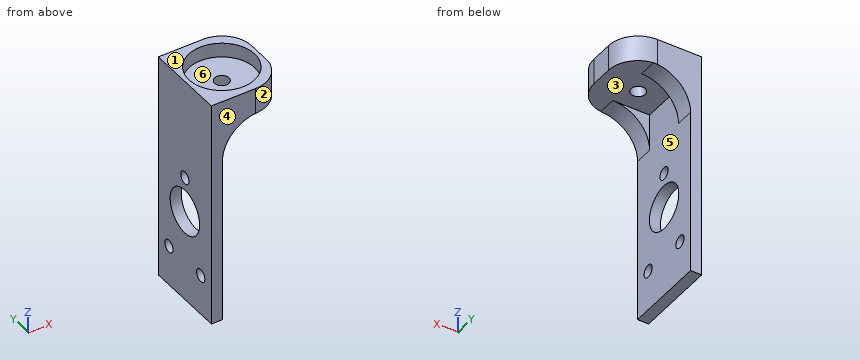
```python
from build123d import *

# Parameters (mm, degrees)
SKETCH1_W                 = 3.81
SKETCH1_H                 = 78.74
SKETCH1_W_2               = 21.59
SKETCH1_H_2               = 8.89
BOSS_EXTRUDE1_DEPTH       = 27.94
SKETCH2_R                 = 11.303
CUT_EXTRUDE1_DEPTH        = 4.953
F_8_CLEARANCE_HOLE1_D     = 4.9149
CUT_EXTRUDE4_REACH        = 88.295
SKETCH5_R                 = 7.747
F_6_CLEARANCE_HOLE1_D     = 4.3053
F_6_CLEARANCE_HOLE1_DEPTH = 3.81
FILLET1_DEPTH             = 6.35
FILLET2_START             = 21.59
FILLET2_DEPTH             = 6.35
FILLET3_R                 = 10.16


with BuildPart() as part:
    # Sketch1 → Boss-Extrude1 (new body)
    with BuildSketch(Plane(origin=(0, 0, 0), x_dir=(1, 0, 0), z_dir=(0, 1, 0))):
        with Locations((1.905, 39.37)):
            Rectangle(SKETCH1_W, SKETCH1_H)
        with Locations((14.605, 4.445)):
            Rectangle(SKETCH1_W_2, SKETCH1_H_2)
    extrude(amount=BOSS_EXTRUDE1_DEPTH)

    # Sketch2 → Cut-Extrude1 (cut)
    with BuildSketch(Plane.XY):
        with Locations((12.7, 13.97)):
            Circle(SKETCH2_R)
    extrude(amount=-CUT_EXTRUDE1_DEPTH, mode=Mode.SUBTRACT)

    # #8 Clearance Hole1 (through all)
    with Locations(Plane.XY.offset(-4.953)):
        with Locations((12.7, 13.97)):
            Hole(F_8_CLEARANCE_HOLE1_D / 2)

    # Sketch5 → Cut-Extrude4 (cut, up to next)
    with BuildSketch(Plane(origin=(3.81, 0, 0), x_dir=(0, 0, -1), z_dir=(1, 0, 0)), mode=Mode.PRIVATE) as cut_extrude4_sk1:
        with Locations((46.99, 13.97)):
            Circle(SKETCH5_R)
    cut_extrude4_tool1 = extrude(cut_extrude4_sk1.sketch, amount=-CUT_EXTRUDE4_REACH, mode=Mode.PRIVATE) & part.part
    # Sketch5 → Cut-Extrude4 (cut, up to next)
    with BuildSketch(Plane(origin=(3.81, 0, 0), x_dir=(0, 0, -1), z_dir=(1, 0, 0)), mode=Mode.PRIVATE) as cut_extrude4_sk2:
        with BuildLine():
            ThreePointArc((54.737, 13.97), (46.99, 21.717), (39.243, 13.97))
            Line((39.243, 13.97), (54.737, 13.97))
        make_face()
    cut_extrude4_tool2 = extrude(cut_extrude4_sk2.sketch, amount=-CUT_EXTRUDE4_REACH, mode=Mode.PRIVATE) & part.part
    # Sketch5 → Cut-Extrude4 (cut, up to next)
    with BuildSketch(Plane(origin=(3.81, 0, 0), x_dir=(0, 0, -1), z_dir=(1, 0, 0)), mode=Mode.PRIVATE) as cut_extrude4_sk3:
        with BuildLine():
            Line((54.737, 13.97), (39.243, 13.97))
            ThreePointArc((39.243, 13.97), (46.99, 6.223), (54.737, 13.97))
        make_face()
    cut_extrude4_tool3 = extrude(cut_extrude4_sk3.sketch, amount=-CUT_EXTRUDE4_REACH, mode=Mode.PRIVATE) & part.part
    add(cut_extrude4_tool1.solids().sort_by_distance((3.81, 13.97, -46.99))[0], mode=Mode.SUBTRACT)
    add(cut_extrude4_tool2.solids().sort_by_distance((3.81, 17.257929, -46.99))[0], mode=Mode.SUBTRACT)
    add(cut_extrude4_tool3.solids().sort_by_distance((3.81, 10.682071, -46.99))[0], mode=Mode.SUBTRACT)

    # #6 Clearance Hole1
    with Locations(Plane(origin=(3.81, 0, 0), x_dir=(0, 0, -1), z_dir=(1, 0, 0))):
        with Locations((34.798, 13.97), (46.99, 13.97), (64.77, 22.352), (64.77, 5.588)):
            Hole(F_6_CLEARANCE_HOLE1_D / 2, depth=F_6_CLEARANCE_HOLE1_DEPTH)

    # Fillet1: read off the stored shape, not the designer's step
    # Fillet1 outline → Fillet1 (add)
    with BuildSketch(Plane(origin=(0, 0, 0), x_dir=(1, 0, 0), z_dir=(0, 1, 0))):
        with BuildLine():
            ThreePointArc((16.51, 8.89), (7.529743879, 12.609743879), (3.81, 21.59))
            Line((3.81, 21.59), (3.81, 8.89))
            Line((3.81, 8.89), (16.51, 8.89))
        make_face()
    extrude(amount=FILLET1_DEPTH)

    # Fillet2: read off the stored shape, not the designer's step
    # Fillet2 outline → Fillet2 (add)
    with BuildSketch(Plane(origin=(0, 0, 0), x_dir=(1, 0, 0), z_dir=(0, 1, 0)).offset(FILLET2_START)):
        with BuildLine():
            ThreePointArc((16.51, 8.89), (7.529743879, 12.609743879), (3.81, 21.59))
            Line((3.81, 21.59), (3.81, 8.89))
            Line((3.81, 8.89), (16.51, 8.89))
        make_face()
    extrude(amount=FILLET2_DEPTH)

    # Fillet3
    fillet3_edges = [part.edges().sort_by_distance(p)[0] for p in [
        (25.4, 0, -4.445),
        (25.4, 27.94, -4.445),
    ]]
    fillet(fillet3_edges, radius=FILLET3_R)


solid = part.part
```
Can you work these out from the model? Positions are in its coordinate system, mm. Face numbers are marked on the shaded views. A direction names the side the tool comes from. Give positions to 0.01 mm unless a question says otherwise; leave off trailing zeros. Write each loop counter-clockwise with the first axis right and the second up, starting at its lowest first coordinate (ties: lowest second). Pieces come first, ordered by that corner, then holes. Notation, with made-up numbers: (20, -17.5) -> (39, -17.5) arc R20 ccw to (39, -6.5) -> close; hole circle Ø1 at (62.5, 49). An arc over 180 degrees is marked (long way). One line per item, written item: value.
Q1. Imagine slicing it at D-D on x = 14. Please give me the cut outline in (y, z).
Results found:
outline: (0, -9.14) -> (6.35, -9.14) -> (6.35, -8.89) -> (11.88, -8.89) -> (11.88, -4.95) -> (2.74, -4.95) -> (2.74, 0) -> (0, 0) -> close; (16.06, -8.89) -> (21.59, -8.89) -> (21.59, -9.14) -> (27.94, -9.14) -> (27.94, 0) -> (25.2, 0) -> (25.2, -4.95) -> (16.06, -4.95) -> close
Q2. Please list where these lines run through material, in increasing order: line 1 (Y direction, x = 2.55, z = -64.77); line 2 (Z direction, x = 3.75, y = 14.75); line 3 (X direction, y = 26.5, z = -65). Write a range as [from, to].
Results found:
line 1: y = [0, 3.44], [7.74, 20.2], [24.5, 27.94]
line 2: z = [-78.74, -54.7], [-39.28, -36.8], [-32.79, -4.95]
line 3: x = [0, 3.81]
Q3. Imagine slicing it at B-B on z = -46.99. Please give me the cut outline in (x, y).
Results found:
outline: (0, 0) -> (3.81, 0) -> (3.81, 6.22) -> (0, 6.22) -> close; (0, 21.72) -> (3.81, 21.72) -> (3.81, 27.94) -> (0, 27.94) -> close
Q4. For P1, Ø10, axis at x = 8.5, z = -16.5, coming from the +Y side; P2, Ø11.5, axis at x = 14, y = 11, coming from the +Z side; P3, Ø11, axis at x = 11.5, y = 17, coming from the -Z side, each with a flat end and sliding along its axis, tell me the tip position at first contact or that it passes through.
Results found:
P1: stops at y = 27.94
P2: stops at z = -4.95
P3: stops at z = -11.76
Q5. We'd pull the mould along Y, two halves only. Please class the marked faces 1, 2 and 3: +Y half, -Y half, draft (parallel to the pull), parting line (faces both ways), or undercut.
Results found:
face 1: draft
face 2: -Y half
face 3: undercut
Q6. Imagine slicing it at A-A on z = -64.77. Please give me the cut outline in (x, y).
Results found:
outline: (0, 0) -> (3.81, 0) -> (3.81, 3.44) -> (0, 3.44) -> close; (0, 7.74) -> (3.81, 7.74) -> (3.81, 20.2) -> (0, 20.2) -> close; (0, 24.5) -> (3.81, 24.5) -> (3.81, 27.94) -> (0, 27.94) -> close
Q7. Imagine slicing it at C-C on y = 8.75. Please give me the cut outline in (x, z).
Results found:
outline: (0, -78.74) -> (3.81, -78.74) -> (3.81, -52.71) -> (0, -52.71) -> close; (0, -41.27) -> (3.81, -41.27) -> (3.81, -8.89) -> (25.3, -8.89) -> (25.3, 0) -> (22.73, 0) -> (22.73, -4.95) -> (2.67, -4.95) -> (2.67, 0) -> (0, 0) -> close
Q8. Which directions (+Z, -Z, +X, -X, +Y, -Y) give clear straight access to the entire face, cutting with the end or side of a thin tool? Please do the marked faces 4, 5 and 6.
Results found:
face 4: +Z, -Z, +X, -X, -Y
face 5: -Z, +X
face 6: +Z
